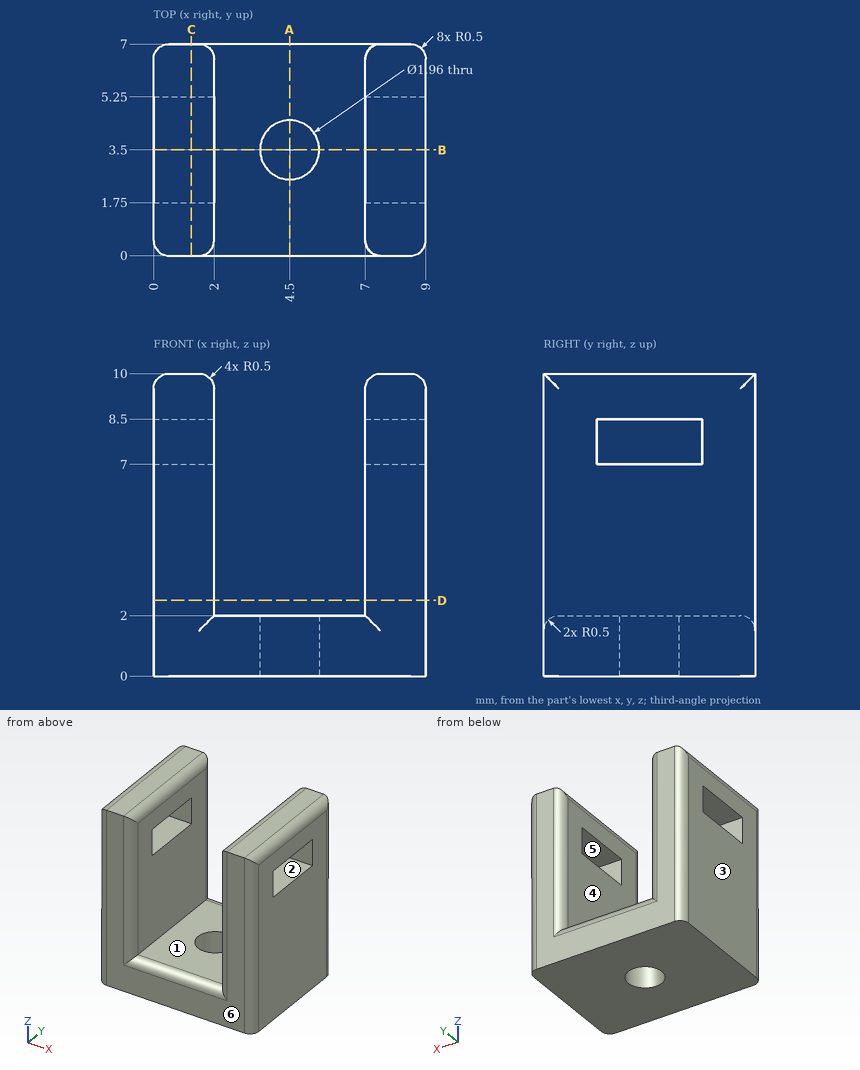
Drawing for the job (mm, zero at the part's lowest x, y, z). A direction names the side the tool comes from. Give positions to 0.01 mm unless a question says otherwise; leave off trailing zeros. Write each loop counter-clockwise with the first axis right and the second up, starting at its lowest first coordinate (ties: lowest second). Pieces come first, ordered by that corner, then holes. Notation, with made-up numbers: M 16,86.5 L 26,86.5 A15 ccw 26,90.5 Z; hole C -17,59 d10. An arc over 180 degrees is marked long. Return JSON: item names as keys, results as strings. Group by question number.
(1) Band-saw the part on C-C (x = 1.25). Give the cut face in (y, z).
(2) Mould opens along Y. For the marked faces 4, 5 and 6 say: pulls with the +Y half, pulls with the -Y half, needs draft (parallel to the pull), parting line crosses it, or undercut.
(3) Band-saw the part on B-B (y = 3.5). Give the cut face in (x, z).
(4) Drill centre lines: L1, parallel to Z at x = 7.75, y = 4; L2, parallel to Y at x = 4.5, z = 1.35; L3, parallel to X at y = 2, z = 5.5. Where is each one in solid material? Low to high. Write a range as [from, to].
(5) 3-axis set-ups, long thin cutter, end or side, ignore diameter. For the marked faces 1, 2 and 3: which of +Z, -Z, +X, -X, +Y, -Y reach the whole face in a straight line?
(6) Band-saw the part on D-D (z = 2.5). Give the cut face in (x, y).
(7) Band-saw the part on A-A (x = 4.5). Give the cut face in (y, z), and give its area (3 significant figures).
(8) Flat gauge pin, fed straight in: pin 1 Ø1.5 at (x, y) = (3.5, 4.5) entering from +Z. Where does the tip first touch, or does it go through?
Entries:
{
 "1": {"outline": "M 0,0 L 7,0 L 7,10 L 0,10 Z; hole M 1.75,7 L 5.25,7 L 5.25,8.5 L 1.75,8.5 Z"},
 "2": {"face 4": "needs draft", "face 5": "undercut", "face 6": "pulls with the -Y half"},
 "3": {"outline": "M 0,0 L 3.52,0 L 3.52,2 L 2,2 L 2,7 L 0,7 Z; M 0,8.5 L 2,8.5 L 2,9.5 A0.5 ccw 1.5,10 L 0.5,10 A0.5 ccw 0,9.5 Z; M 5.48,0 L 9,0 L 9,7 L 7,7 L 7,2 L 5.48,2 Z; M 7,8.5 L 9,8.5 L 9,9.5 A0.5 ccw 8.5,10 L 7.5,10 A0.5 ccw 7,9.5 Z"},
 "4": {"L1": "z = [0, 7], [8.5, 10]", "L2": "y = [0, 2.52], [4.48, 7]", "L3": "x = [0, 2], [7, 9]"},
 "5": {"face 1": "+Z, +Y, -Y", "face 2": "+X, -X", "face 3": "+Z, -Z, -X, +Y, -Y"},
 "6": {"outline": "M 0,0.5 A0.5 ccw 0.5,0 L 1.5,0 A0.5 ccw 2,0.5 L 2,6.5 A0.5 ccw 1.5,7 L 0.5,7 A0.5 ccw 0,6.5 Z; M 7,0.5 A0.5 ccw 7.5,0 L 8.5,0 A0.5 ccw 9,0.5 L 9,6.5 A0.5 ccw 8.5,7 L 7.5,7 A0.5 ccw 7,6.5 Z"},
 "7": {"outline": "M 0,0 L 2.52,0 L 2.52,2 L 0.5,2 A0.5 ccw 0,1.5 Z; M 4.48,0 L 7,0 L 7,1.5 A0.5 ccw 6.5,2 L 4.48,2 Z", "area": "9.97 mm^2"},
 "8": {"pin 1": "stops at z = 2"}
}
